The model under review builds one solid part; all positions refer to its coordinate system, in mm. Face numbers are marked on the shaded views. A direction names the side the tool comes from. Round coordinates to 2 decimals unless told otherwise and drop trailing zeros. Write each loop counter-clockwise with the first axis right and the second up, starting at its lowest first coordinate (ties: lowest second). Pieces come first, ordered by that corner, then holes. Notation, with made-up numbers: (-15, -7.5) -> (-9, -7.5) arc R15 cw to (-9, 8.5) -> close; hole circle Ø4 at (44.25, -6). An arc over 180 degrees is marked (long way). Return JSON: item names as keys, results as strings. Group by question number.
1. Take a section at B-B, the plane z = 1.9. Write out the cut boundary in (x, y), then the cut area to 3 significant figures.
2. For line 1 along X through (y, z) = (15.75, 0.85); line 2 along Y through (x, z) = (20, 3.7); line 3 along Y through (x, z) = (14.5, 1.05), list the stretches that pass through material, from the lowest coordinate up. Write a range as from..to.
3. Tool access review of the marked faces 1, 2 and 3: name each direction out of +Z, -Z, +X, -X, +Y, -Y from which nothing blocks a thin tool from reaching the whole face with its end or side.
4. Take a section at D-D, the plane z = 3.45. Write out the cut boundary in (x, y).
5. Mouldability with a two-part tool opening along X and no side actions: class the marked faces 4, 5 and 6 as pulls with the +X half, pulls with the -X half, needs draft (parallel to the pull), parting line crosses it, or undercut.
6. Take a section at C-C, the plane x = 18.5. Write out the cut boundary in (y, z).
7. Take a section at A-A, the plane y = 17. Write out the cut boundary in (x, z), then the cut area to 3 significant figures.
Autodesk Fusion 360 part; units mm, degrees
sketch "Sketch1" plane through (0, 0, 0) normal (0, 0, 1) x (1, 0, 0)
  line L0 (5.2435, 4.6143) -> (24.2435, 4.6143)
  line L1 (24.2435, 4.6143) -> (24.2435, 23.6143)
  line L2 (24.2435, 23.6143) -> (5.2435, 23.6143)
  line L3 (5.2435, 23.6143) -> (5.2435, 4.6143)
  line L4 (5.2435, 23.6143) -> (24.2435, 4.6143) construction
  line L5 (24.2435, 23.6143) -> (5.2435, 4.6143) construction
  line L6 (5.2435, 4.6143) -> (10.3435, 4.6143) construction
  line L7 (5.2435, 4.6143) -> (7.7935, 4.6143) construction
  line L8 (7.7935, 4.6143) -> (7.7935, 23.6143) construction
  line L9 (7.7935, 7.1643) -> (21.6935, 7.1643)
  line L10 (21.6935, 7.1643) -> (21.6935, 21.0643)
  line L11 (21.6935, 21.0643) -> (7.7935, 21.0643)
  line L12 (7.7935, 21.0643) -> (7.7935, 7.1643)
  dimension "d1" = 19
  dimension "d2" = 19
  dimension "d4" = 2.55
  dimension "d5" = 13.9
  dimension "d6" = 13.9
extrude "Extrude1" add sketch "Sketch1" along normal blind 4
sketch "Sketch2" plane through (0, 21.0643, 0) normal (0, -1, 0) x (1, 0, 0)
  line L0 (7.7935, 0) -> (21.6935, 0)
  line L1 (21.6935, 0) -> (21.6935, 4)
  line L2 (21.6935, 4) -> (7.7935, 4)
  line L3 (7.7935, 4) -> (7.7935, 0)
  line L4 (14.7435, 0) -> (17.2435, 0) construction
  line L5 (17.2435, 0) -> (12.2435, 0)
  line L6 (12.2435, 0) -> (12.2435, 2.7)
  line L7 (12.2435, 2.7) -> (17.2435, 2.7)
  line L8 (17.2435, 2.7) -> (17.2435, 0)
  dimension "d9" = 2.5
  dimension "d10" = 5
  dimension "d11" = 2.7
extrude "Extrude2" add sketch "Sketch2" along normal blind 0.5 contours L0 L5 L6 L7 L8
extrude "Extrude3" cut 1 faces at (13.9102, 20.5643, 0.9) along direction (0, 1, 0) blind 1
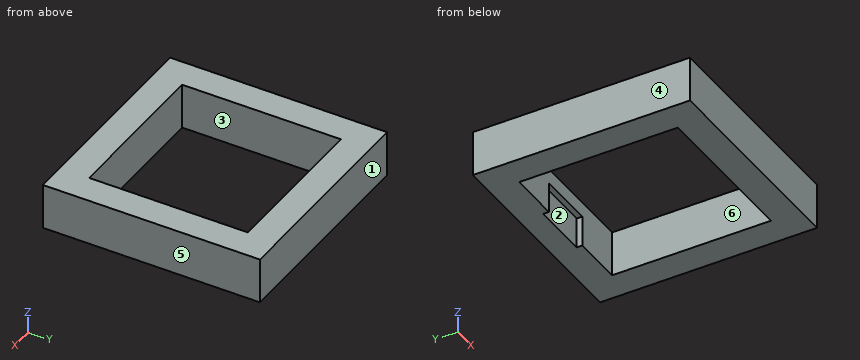
Output:
{
 "1": {"outline": "(5.24, 4.61) -> (24.24, 4.61) -> (24.24, 23.61) -> (5.24, 23.61) -> close; hole (7.79, 7.16) -> (21.69, 7.16) -> (21.69, 21.06) -> (17.24, 21.06) -> (17.24, 21.56) -> (12.24, 21.56) -> (12.24, 21.06) -> (7.79, 21.06) -> close", "area": "165 mm^2"},
 "2": {"line 1": "x = 5.24..7.79, 21.69..24.24", "line 2": "y = 4.61..7.16, 21.06..23.61", "line 3": "y = 4.61..7.16, 21.56..23.61"},
 "3": {"face 1": "+Z, -Z, +X, -X, +Y", "face 2": "-Z", "face 3": "+Z, -Z"},
 "4": {"outline": "(5.24, 4.61) -> (24.24, 4.61) -> (24.24, 23.61) -> (5.24, 23.61) -> close; hole (7.79, 7.16) -> (21.69, 7.16) -> (21.69, 21.06) -> (7.79, 21.06) -> close"},
 "5": {"face 4": "pulls with the -X half", "face 5": "pulls with the +X half", "face 6": "undercut"},
 "6": {"outline": "(4.61, 0) -> (7.16, 0) -> (7.16, 4) -> (4.61, 4) -> close; (21.06, 0) -> (23.61, 0) -> (23.61, 4) -> (21.06, 4) -> close"},
 "7": {"outline": "(5.24, 0) -> (7.79, 0) -> (7.79, 4) -> (5.24, 4) -> close; (21.69, 0) -> (24.24, 0) -> (24.24, 4) -> (21.69, 4) -> close", "area": "20.4 mm^2"}
}
